Design review of the part shown in the three views and the two pictorial views. Dimensions are in mm from the part's minimum x, y and z. A direction names the side the tool comes from. Coordinates: 2 decimals unless noted, no trailing zeros. Loops run counter-clockwise (first coordinate to the right, second up) from the corner with the lowest first, then second, coordinate; pieces in that order, holes last. Notation, with made-up numbers: (9, 62.5) -> (49, 62.5) arc R8 cw to (49, 70.5) -> close; hole circle Ø7 at (46, 73). An arc over 180 degrees is marked (long way). One line per item, written item: value. Start each with the question number.
1. Add section A-A on z = 2.5. Write out the cut boundary in (x, y).
2. Add section B-B on y = 11. Write out the cut boundary in (x, z).
3. Insertion check: pin 1 (2.5 mm diameter, centred on y = 22, z = 3.5, fed in from -X); pin 2 (2.5 mm diameter, centred on x = 32, y = 2, fed in from -Z); pin 3 (1.5 mm diameter, centred on y = 23.5, z = 3, fed in from +X); pin 4 (1.5 mm diameter, centred on x = 9.5, z = 3.5, fed in from -Y). Each pin has a flat end and moves straight along its axis. Give the tip position at first contact, or say it passes through.
4. For probe 1 along Y at (x, z) = (32, 0.7); probe 2 along X at (y, z) = (13, 2.7); probe 3 along Z at (x, y) = (7.5, 26), list the stretches that pass through material, from the lowest coordinate up.
5. Machinability: for the marked faces 4, 5 and 6, which of the approach directions +Z, -Z, +X, -X, +Y, -Y give a long, thin tool a straight path to every point of the face, cutting with its end or side? Answer none if there is none.
6. Draft analysis for pull direction Y (two halves, no side actions). For the marked faces 1, 2 and 3, state which applies: pulls with the +Y half, pulls with the -Y half, needs draft (parallel to the pull), parting line crosses it, or undercut.
7. Add section D-D on x = 16.5. Write out the cut boundary in (y, z).
8. Add section C-C on x = 21.5. Write out the cut boundary in (y, z), plus the area to 3 significant figures.
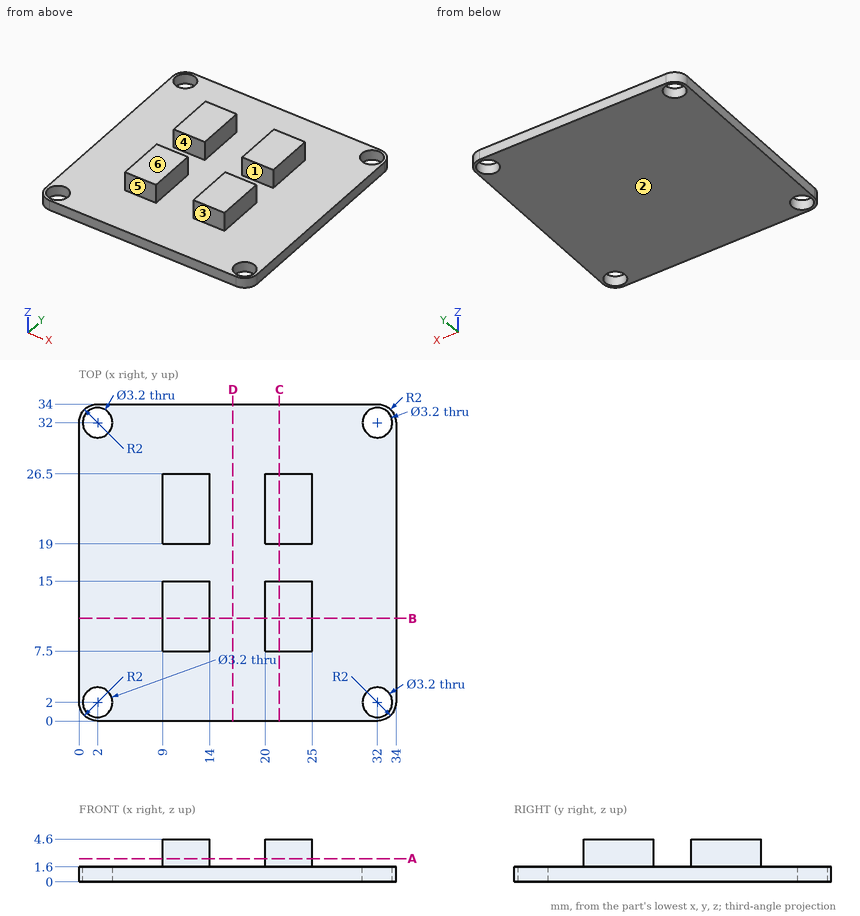
Worked answers:
1. outline: (9, 7.5) -> (14, 7.5) -> (14, 15) -> (9, 15) -> close; (9, 19) -> (14, 19) -> (14, 26.5) -> (9, 26.5) -> close; (20, 7.5) -> (25, 7.5) -> (25, 15) -> (20, 15) -> close; (20, 19) -> (25, 19) -> (25, 26.5) -> (20, 26.5) -> close
2. outline: (0, 0) -> (34, 0) -> (34, 1.6) -> (25, 1.6) -> (25, 4.6) -> (20, 4.6) -> (20, 1.6) -> (14, 1.6) -> (14, 4.6) -> (9, 4.6) -> (9, 1.6) -> (0, 1.6) -> close
3. pin 1: stops at x = 9
3. pin 2: passes through
3. pin 3: stops at x = 25
3. pin 4: stops at y = 7.5
4. probe 1: y = 0 to 0.4, 3.6 to 30.4, 33.6 to 34
4. probe 2: x = 9 to 14, 20 to 25
4. probe 3: z = 0 to 1.6
5. face 4: +Z, +X, -X
5. face 5: +Z, +X, -X, -Y
5. face 6: +Z, +X, -X, +Y, -Y
6. face 1: undercut
6. face 2: needs draft
6. face 3: pulls with the -Y half
7. outline: (0, 0) -> (34, 0) -> (34, 1.6) -> (0, 1.6) -> close
8. outline: (0, 0) -> (34, 0) -> (34, 1.6) -> (26.5, 1.6) -> (26.5, 4.6) -> (19, 4.6) -> (19, 1.6) -> (15, 1.6) -> (15, 4.6) -> (7.5, 4.6) -> (7.5, 1.6) -> (0, 1.6) -> close
8. area: 99.4 mm²
